Input: dimensioned drawing with shaded views. Units: mm. Origin: part minimum x, y, z. A direction names the side the tool comes from. Round coordinates to 2 decimals unless told otherwise and drop trailing zeros. Loops run counter-clockwise (first coordinate to the right, second up) from the corner with the lowest first, then second, coordinate; pieces in that order, holes last. Notation, with made-up numbers: (-3.5, 33) -> (1.5, 33) arc R5 cw to (1.5, 37) -> close; hole circle Ø4 at (81.25, -35). An arc over 180 degrees is marked (long way). Answer as a JSON object with one key per item and string values.
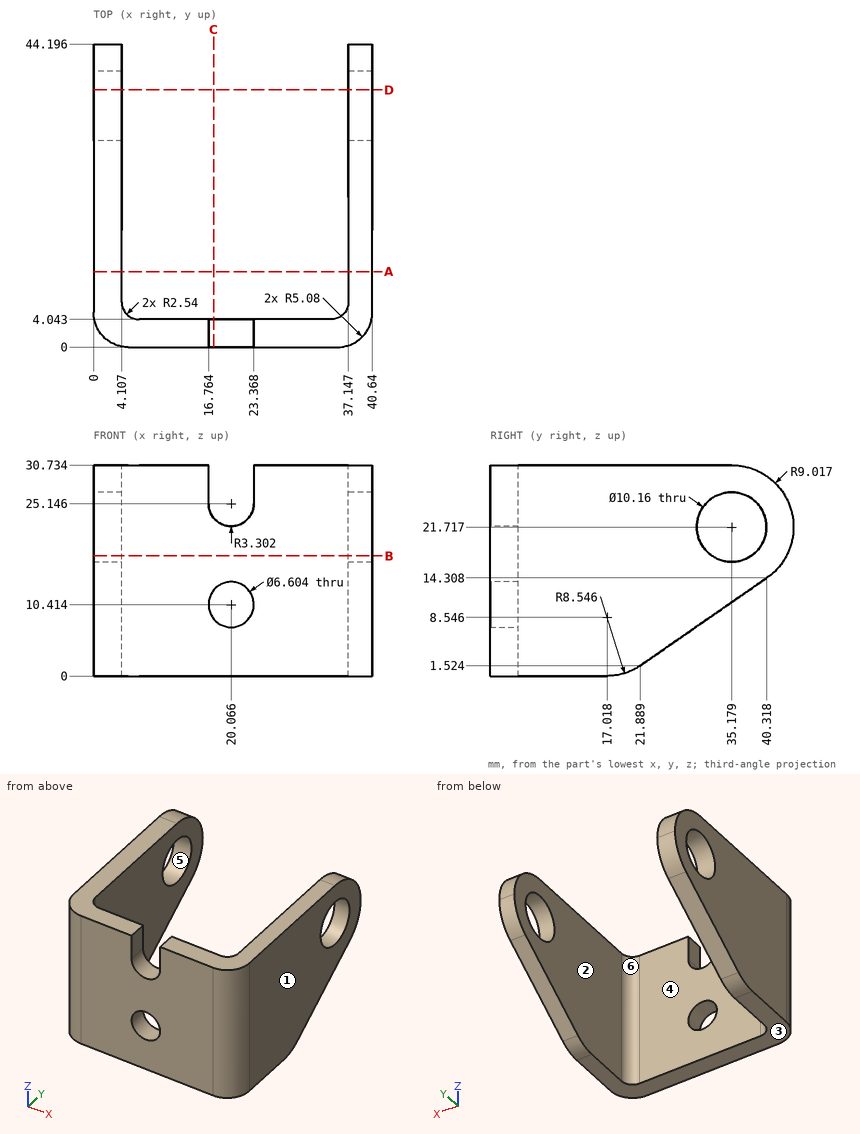
1) Contact query for flat-ended pins moving along their axis: P1, Ø2, axis at y = 3, z = 29, coming from the -X side; P2, Ø8, axis at x = 10, y = 30, coming from the -Z side; P3, Ø4.5, axis at y = 1, z = 27.5, coming from the +X side. Output: stop coordinate, or through.
Output:
{"P1": "stops at x = 0.12", "P2": "passes through", "P3": "stops at x = 40.3"}
2) Section C-C, the plane x = 17.5. Output: boundary loops of the cut face in (y, z).
Output:
{"outline": "(0, 0) -> (4.04, 0) -> (4.04, 8.34) -> (0, 8.34) -> close; (0, 12.49) -> (4.04, 12.49) -> (4.04, 23.07) -> (0, 23.07) -> close"}
3) Section B-B, the plane z = 17.5. Output: boundary loops of the cut face in (x, y), plus the area to 3 significant figures.
Output:
{"outline": "(0, 5.08) arc R5.08 ccw to (5.08, 0) -> (35.56, 0) arc R5.08 ccw to (40.64, 5.08) -> (40.64, 32.35) -> (37.15, 32.35) -> (37.15, 6.58) arc R2.54 cw to (34.61, 4.04) -> (6.65, 4.04) arc R2.54 cw to (4.11, 6.58) -> (4.11, 32.35) -> (0, 32.35) -> close; (0, 38.01) -> (4.11, 38.01) -> (4.11, 43.15) -> (0, 43.15) -> close; (37.15, 38.01) -> (40.64, 38.01) -> (40.64, 43.15) -> (37.15, 43.15) -> close", "area": "410 mm^2"}
4) Ray query, probe 1 along X at (y, z) = (28, 19); probe 2 along Y at (x, z) = (31.5, 29); probe 3 along X at (y, z) = (2.5, 7) (1 decimal). Return the intervals inside material, ascending.
Output:
{"probe 1": "x = 0 to 4.11, 37.15 to 40.64", "probe 2": "y = 0 to 4.04", "probe 3": "x = 0.7 to 39.9"}
5) Reachability of the marked faces 5 and 6 from +Z, -Z, +X, -X, +Y, -Y: full face, straight path, thin tool, end or side. Return the list, or none.
Output:
{"face 5": "+X, -X", "face 6": "+Z, -Z, +Y"}
6) Section A-A, the plane y = 11. Output: boundary loops of the cut face in (x, z).
Output:
{"outline": "(0, 0) -> (4.11, 0) -> (4.11, 30.73) -> (0, 30.73) -> close; (37.15, 0) -> (40.64, 0) -> (40.64, 30.73) -> (37.15, 30.73) -> close"}
7) Draft query along X for the marked faces 1, 2, 3 and 4. Return one class per face: +X half, -X half, draft (parallel to the pull), parting line (faces both ways), or undercut.
Output:
{"face 1": "+X half", "face 2": "undercut", "face 3": "draft", "face 4": "undercut"}
8) Section D-D, the plane y = 37.5. Output: boundary loops of the cut face in (x, z) (1 decimal).
Output:
{"outline": "(0, 12.4) -> (4.1, 12.4) -> (4.1, 17.2) -> (0, 17.2) -> close; (0, 26.2) -> (4.1, 26.2) -> (4.1, 30.4) -> (0, 30.4) -> close; (37.1, 12.4) -> (40.6, 12.4) -> (40.6, 17.2) -> (37.1, 17.2) -> close; (37.1, 26.2) -> (40.6, 26.2) -> (40.6, 30.4) -> (37.1, 30.4) -> close"}
